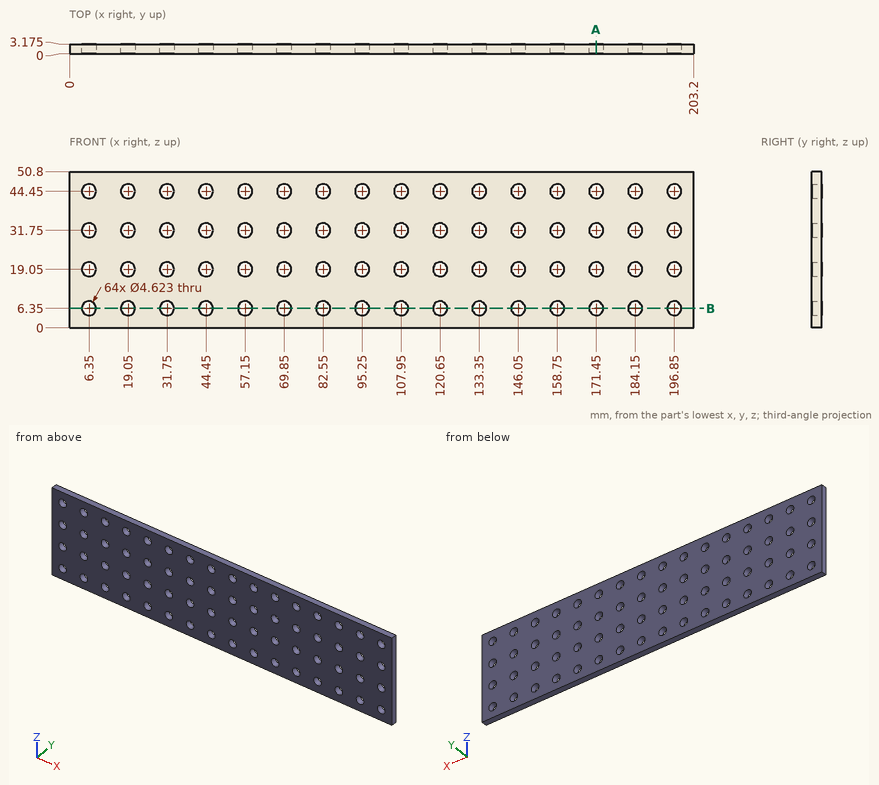
The figure shows three views and two pictorial views of one solid part (mm, origin at its lowest corner). Answer the questions. Coordinates: 2 decimals unless noted, no trailing zeros. Write each loop counter-clockwise with the first axis right and the second up, starting at its lowest first coordinate (ties: lowest second). Pieces come first, ordered by that corner, then holes.
1. Consider line 1 along Z through (x, y) = (171.45, 2.5); line 2 along Z through (x, y) = (170, 1.9). Determine where each line is inside the solid, lowest interval first.
Results list:
line 1: z = 0 to 4.04, 8.66 to 16.74, 21.36 to 29.44, 34.06 to 42.14, 46.76 to 50.8
line 2: z = 0 to 4.55, 8.15 to 17.25, 20.85 to 29.95, 33.55 to 42.65, 46.25 to 50.8
2. A flat-ended cylindrical pin translates along its axis: pin 1 (7.5 mm diameter, centred on x = 107.95, z = 44.45, fed in from -Y). Find the tip coordinate at first contact, or state that the pin passes through.
Results list:
pin 1: stops at y = 0
3. The part is cut by section B-B, the plane z = 6.35. State how many separate pieces and enclosed holes the cut face has, and give its area (3 significant figures).
Results list:
separate pieces: 17
enclosed holes: 0
area: 410 mm2
4. The part is cut by section A-A, the plane x = 171.45. Write down the section's boundary in (y, z) (1 decimal).
Results list:
outline: (0, 0) - (3.2, 0) - (3.2, 4) - (0, 4) - close; (0, 8.7) - (3.2, 8.7) - (3.2, 16.7) - (0, 16.7) - close; (0, 21.4) - (3.2, 21.4) - (3.2, 29.4) - (0, 29.4) - close; (0, 34.1) - (3.2, 34.1) - (3.2, 42.1) - (0, 42.1) - close; (0, 46.8) - (3.2, 46.8) - (3.2, 50.8) - (0, 50.8) - close
